from build123d import *

# Parameters (mm, degrees)
F1_DEPTH     = 63.5
F0_W         = 25.4
F0_H         = 9.398
F2_DEPTH     = 25.4
F3_DEPTH     = 7.9375
F5_R         = 6.35
F6_T1_DEPTH  = 41.275
F6_T3_DEPTH  = 69.85
F6_T5_DEPTH  = 49.2125
F6_T7_DEPTH  = 49.2125
F6_T9_DEPTH  = 31.75
F6_T11_DEPTH = 31.75
F6_T13_DEPTH = 31.877
F6_T16_ANGLE = 90
F6_T18_ANGLE = 90
F6_T20_ANGLE = 90
F6_T22_ANGLE = 90
F6_T24_ANGLE = 90
F6_T26_ANGLE = 90


# Not quite as in the source:
# - a fillet or chamfer that OpenCascade refuses, or shapes differently, is made with other operations: its cross-section is extruded or revolved along the edge and cut away or added


with BuildPart() as f1:
    # F0 (on Front) → F1 (new body, symmetric)
    with BuildSketch(Plane.XZ):
        Polygon((-41.275, 9.525), (-41.275, -9.525), (41.275, -9.525), (41.275, 9.525), (22.225, 9.525), align=None)
    extrude(amount=F1_DEPTH, both=True)

    # F0 (on Front) → F2 (join, symmetric)
    with BuildSketch(Plane.XZ):
        with BuildLine():
            Line((22.225, 9.525), (41.275, 9.525))
            Line((41.275, 9.525), (41.275, 41.402))
            ThreePointArc((41.275, 41.402), (45.9246798487, 52.6273201513), (57.15, 57.277))
            Line((57.15, 57.277), (60.325, 57.277))
            Line((60.325, 57.277), (60.325, 66.675))
            Line((60.325, 66.675), (85.725, 66.675))
            Line((85.725, 66.675), (85.725, 76.327))
            Line((85.725, 76.327), (57.15, 76.327))
            ThreePointArc((57.15, 76.327), (32.4542956671, 66.0977043329), (22.225, 41.402))
            Line((22.225, 41.402), (22.225, 9.525))
        make_face()
        with Locations((73.025, 61.976)):
            Rectangle(F0_W, F0_H)
    extrude(amount=F2_DEPTH, both=True)

    # F0 (on Front) → F3 (join, symmetric)
    with BuildSketch(Plane.XZ):
        with BuildLine():
            add(Edge.make_bspline(
                [(-41.275, 9.525), (-40.9312584529, 49.0607376979), (0, 82.7295482159), (57.15, 76.327)],
                knots=[0, 0, 0, 0, 118.9537213752, 118.9537213752, 118.9537213752, 118.9537213752], degree=3))
            Line((-41.275, 9.525), (22.225, 9.525))
            Line((22.225, 9.525), (22.225, 41.402))
            ThreePointArc((22.225, 41.402), (32.4542956671, 66.0977043329), (57.15, 76.327))
        make_face()
    extrude(amount=F3_DEPTH, both=True)

    # F0 (on Front) → F4 (revolve)
    with BuildSketch(Plane.XZ):
        Polygon((111.125, 66.675), (85.725, 66.675), (85.725, 57.277), (85.725, 34.925), (111.125, 34.925), align=None)
    revolve(axis=Axis((85.725, 0, 55.626), (0, 0, 1)))

    # F5
    f5_edges = [f1.edges().sort_by_distance(p)[0] for p in [
        (41.275, 63.5, 0),
        (-41.275, 63.5, 0),
        (-41.275, -63.5, 0),
        (41.275, -63.5, 0),
    ]]
    fillet(f5_edges, radius=F5_R)

    # F6: fillet of radius 5.08 on 16 edges, made by hand

    # F6_s2 → F6_t1 (cut)
    with BuildSketch(Plane.YZ.offset(57.15)):
        with BuildLine():
            ThreePointArc((25.4, 71.247), (23.9121024484, 74.8391024484), (20.32, 76.327))
            Line((20.32, 76.327), (25.4, 76.327))
            Line((25.4, 76.327), (25.4, 71.247))
        make_face()
        with BuildLine():
            ThreePointArc((-25.4, 71.247), (-23.9121024484, 74.8391024484), (-20.32, 76.327))
            Line((-20.32, 76.327), (-25.4, 76.327))
            Line((-25.4, 76.327), (-25.4, 71.247))
        make_face()
    extrude(amount=F6_T1_DEPTH, mode=Mode.SUBTRACT)

    # F6_s4 → F6_t3 (cut)
    with BuildSketch(Plane.YZ.offset(-34.925)):
        with BuildLine():
            ThreePointArc((-58.42, 9.525), (-62.0121024484, 8.0371024484), (-63.5, 4.445))
            Line((-63.5, 4.445), (-63.5, 9.525))
            Line((-63.5, 9.525), (-58.42, 9.525))
        make_face()
        with BuildLine():
            ThreePointArc((58.42, 9.525), (62.0121024484, 8.0371024484), (63.5, 4.445))
            Line((63.5, 4.445), (63.5, 9.525))
            Line((63.5, 9.525), (58.42, 9.525))
        make_face()
    extrude(amount=F6_T3_DEPTH, mode=Mode.SUBTRACT)

    # F6_s6 → F6_t5 (cut)
    with BuildSketch(Plane.XZ.offset(-57.15)):
        with BuildLine():
            ThreePointArc((-41.275, 4.445), (-39.7871024484, 8.0371024484), (-36.195, 9.525))
            Line((-36.195, 9.525), (-41.275, 9.525))
            Line((-41.275, 9.525), (-41.275, 4.445))
        make_face()
    extrude(amount=F6_T5_DEPTH, mode=Mode.SUBTRACT)

    # F6_s8 → F6_t7 (cut)
    with BuildSketch(Plane.XZ.offset(7.9375)):
        with BuildLine():
            ThreePointArc((-41.275, 4.445), (-39.7871024484, 8.0371024484), (-36.195, 9.525))
            Line((-36.195, 9.525), (-41.275, 9.525))
            Line((-41.275, 9.525), (-41.275, 4.445))
        make_face()
    extrude(amount=F6_T7_DEPTH, mode=Mode.SUBTRACT)

    # F6_s10 → F6_t9 (cut)
    with BuildSketch(Plane.XZ.offset(-57.15)):
        with BuildLine():
            ThreePointArc((36.195, 9.525), (39.7871024484, 8.0371024484), (41.275, 4.445))
            Line((41.275, 4.445), (41.275, 9.525))
            Line((41.275, 9.525), (36.195, 9.525))
        make_face()
    extrude(amount=F6_T9_DEPTH, mode=Mode.SUBTRACT)

    # F6_s12 → F6_t11 (cut)
    with BuildSketch(Plane.XZ.offset(25.4)):
        with BuildLine():
            ThreePointArc((36.195, 9.525), (39.7871024484, 8.0371024484), (41.275, 4.445))
            Line((41.275, 4.445), (41.275, 9.525))
            Line((41.275, 9.525), (36.195, 9.525))
        make_face()
    extrude(amount=F6_T11_DEPTH, mode=Mode.SUBTRACT)

    # F6_s14 → F6_t13 (cut)
    with BuildSketch(Plane.XY.offset(9.525)):
        with BuildLine():
            ThreePointArc((22.225, 20.32), (23.7128975516, 23.9121024484), (27.305, 25.4))
            Line((27.305, 25.4), (22.225, 25.4))
            Line((22.225, 25.4), (22.225, 20.32))
        make_face()
        with BuildLine():
            ThreePointArc((22.225, -20.32), (23.7128975516, -23.9121024484), (27.305, -25.4))
            Line((27.305, -25.4), (22.225, -25.4))
            Line((22.225, -25.4), (22.225, -20.32))
        make_face()
    extrude(amount=F6_T13_DEPTH, mode=Mode.SUBTRACT)

    # F6_s15 → F6_t16 (revolve, cut)
    with BuildSketch(Plane.XZ.offset(-57.15)):
        with BuildLine():
            ThreePointArc((-41.275, 4.445), (-39.7871024484, 8.0371024484), (-36.195, 9.525))
            Line((-36.195, 9.525), (-41.275, 9.525))
            Line((-41.275, 9.525), (-41.275, 4.445))
        make_face()
    revolve(axis=Axis((-34.925, 57.15, 9.525), (0, 0, -1)), revolution_arc=F6_T16_ANGLE, mode=Mode.SUBTRACT)

    # F6_s17 → F6_t18 (revolve, cut)
    with BuildSketch(Plane.XZ.offset(57.15)):
        with BuildLine():
            ThreePointArc((-41.275, 4.445), (-39.7871024484, 8.0371024484), (-36.195, 9.525))
            Line((-36.195, 9.525), (-41.275, 9.525))
            Line((-41.275, 9.525), (-41.275, 4.445))
        make_face()
    revolve(axis=Axis((-34.925, -57.15, 9.525), (0, 0, 1)), revolution_arc=F6_T18_ANGLE, mode=Mode.SUBTRACT)

    # F6_s19 → F6_t20 (revolve, cut)
    with BuildSketch(Plane.YZ.offset(34.925)):
        with BuildLine():
            ThreePointArc((58.42, 9.525), (62.0121024484, 8.0371024484), (63.5, 4.445))
            Line((63.5, 4.445), (63.5, 9.525))
            Line((63.5, 9.525), (58.42, 9.525))
        make_face()
    revolve(axis=Axis((34.925, 57.15, 9.525), (0, 0, -1)), revolution_arc=F6_T20_ANGLE, mode=Mode.SUBTRACT)

    # F6_s21 → F6_t22 (revolve, cut)
    with BuildSketch(Plane.YZ.offset(34.925)):
        with BuildLine():
            ThreePointArc((-58.42, 9.525), (-62.0121024484, 8.0371024484), (-63.5, 4.445))
            Line((-63.5, 4.445), (-63.5, 9.525))
            Line((-63.5, 9.525), (-58.42, 9.525))
        make_face()
    revolve(axis=Axis((34.925, -57.15, 9.525), (0, 0, 1)), revolution_arc=F6_T22_ANGLE, mode=Mode.SUBTRACT)

    # F6_s23 → F6_t24 (revolve, cut)
    with BuildSketch(Plane.YZ.offset(57.15)):
        with BuildLine():
            ThreePointArc((25.4, 71.247), (23.9121024484, 74.8391024484), (20.32, 76.327))
            Line((20.32, 76.327), (25.4, 76.327))
            Line((25.4, 76.327), (25.4, 71.247))
        make_face()
    revolve(axis=Axis((57.15, 25.4, 41.402), (0, -1, 0)), revolution_arc=F6_T24_ANGLE, mode=Mode.SUBTRACT)

    # F6_s25 → F6_t26 (revolve, cut)
    with BuildSketch(Plane.YZ.offset(57.15)):
        with BuildLine():
            ThreePointArc((-25.4, 71.247), (-23.9121024484, 74.8391024484), (-20.32, 76.327))
            Line((-20.32, 76.327), (-25.4, 76.327))
            Line((-25.4, 76.327), (-25.4, 71.247))
        make_face()
    revolve(axis=Axis((57.15, -25.4, 41.402), (0, -1, 0)), revolution_arc=F6_T26_ANGLE, mode=Mode.SUBTRACT)


solid = f1.part
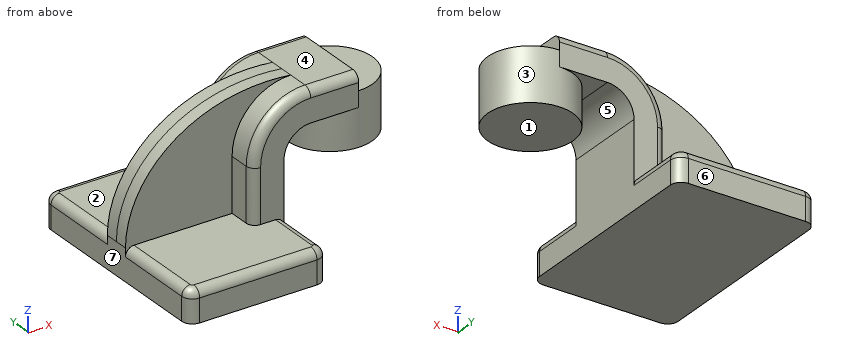
The model under review builds one solid part; all positions refer to its coordinate system, in mm. Face numbers are marked on the shaded views. A direction names the side the tool comes from. Give positions to 0.01 mm unless a question says otherwise; leave off trailing zeros. Loops run counter-clockwise (first coordinate to the right, second up) from the corner with the lowest first, then second, coordinate; pieces in that order, holes last. Notation, with made-up numbers: (67.25, 85.25) -> (96.25, 85.25) arc R30 cw to (96.25, 117.25) -> close; hole circle Ø5 at (60, -36). An arc over 180 degrees is marked (long way). Answer as a JSON object with one key per item and string values. Group by question number.
Q1. Draft analysis for pull direction X (two halves, no side actions). For the marked faces 5, 6 and 7, state which applies: pulls with the +X half, pulls with the -X half, needs draft (parallel to the pull), parting line crosses it, or undercut.
Q2. Tool access review of the marked faces 1, 2, 3 and 4: name each direction out of +Z, -Z, +X, -X, +Y, -Y from which nothing blocks a thin tool from reaching the whole face with its end or side.
Q3. Take a section at A-A (y = -46.5). Write out the cut boundary in (x, z) (3 decimals).
Q4. Wall thickness on line 1 along Z through (x, y) = (25.5, 47.5) (3 decimals); line 2 along Y through (x, z) = (56, 59); line 3 along X through (y, z) = (-19, 11) (3 decimals): over which ranges is each line inside the solid? List them lowest first.
Q5. Take a section at B-B (x = 93). Write out the cut boundary in (y, z) (3 decimals).
Q6. Insertion check: pin 1 (14.5 mm diameter, centred on x = 65, y = 3, fed in from -Z) (3 decimals); pin 2 (1 mm diameter, centred on y = -13.5, z = 42.5, fed in from +X); pin 3 (7.5 mm diameter, centred on y = -9.5, z = 70, fed in from +X); pin 4 (12 mm diameter, centred on y = 37, z = 43.5, fed in from +X). Each pin has a flat end and moves straight along its axis. Give the tip position at first contact, or say it passes through.
Answer below:
{
 "1": {"face 5": "undercut", "face 6": "needs draft", "face 7": "pulls with the -X half"},
 "2": {"face 1": "-Z, +X, +Y, -Y", "face 2": "+Z, -X, +Y", "face 3": "-Z", "face 4": "+Z, +X, +Y, -Y"},
 "3": {"outline": "(-41.275, -9.525) -> (41.275, -9.525) -> (41.275, 4.445) arc R5.08 ccw to (36.195, 9.525) -> (-36.195, 9.525) arc R5.08 ccw to (-41.275, 4.445) -> close"},
 "4": {"line 1": "z = -9.525 to 9.525", "line 2": "y = -25.4 to 25.4", "line 3": "x = 22.225 to 41.275"},
 "5": {"outline": "(-24.336, 34.925) -> (24.336, 34.925) -> (24.336, 66.675) -> (-24.336, 66.675) -> close"},
 "6": {"pin 1": "stops at z = 34.925", "pin 2": "stops at x = 107.55", "pin 3": "stops at x = 109.91", "pin 4": "passes through"}
}
